Part model, mm, in its own coordinate system. Face numbers are marked on the shaded views. Give positions to 0.01 mm unless a question says otherwise; leave off trailing zeros. Write each loop counter-clockwise with the first axis right and the second up, starting at its lowest first coordinate (ties: lowest second). Pieces come first, ordered by that corner, then holes. Notation, with made-up numbers: (88, 80.25) - (147, 80.25) arc R28 ccw to (147, 118.25) - close; hole circle Ø11 at (63, 16). An arc over 180 degrees is marked (long way). Answer as a JSON object with one key per item and string values. Group by question number.
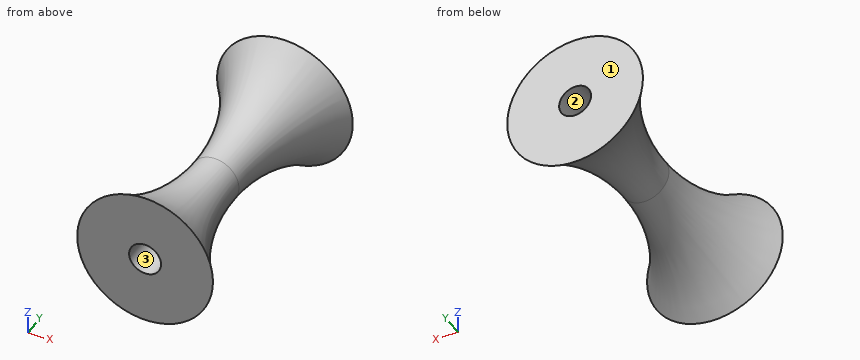
```python
from build123d import *

# Parameters (mm, degrees)
SKETCH1_W          = 3
SKETCH1_H          = 32
SKETCH2_R          = 2
CUT_EXTRUDE1_DEPTH = 35.18332927
CUT_EXTRUDE2_START = -4
SKETCH3_R          = 2.5
CUT_EXTRUDE2_DEPTH = 24
FILLET1_R          = 0.5


with BuildPart() as part:
    # Sketch1 → Revolve1 (revolve)
    with BuildSketch(Plane.XY, mode=Mode.PRIVATE) as revolve1_sk:
        with BuildLine():
            Line((-3, -7e-08), (-3, 16))
            Line((-3, 16), (-8.5, 16))
            ThreePointArc((-8.5, 16), (-4.413382802, 8.459462125), (-3, -7e-08))
        make_face()
        with Locations((-1.5, 0)):
            Rectangle(SKETCH1_W, SKETCH1_H)
        with BuildLine():
            Line((-8.5, -16), (-3, -16))
            Line((-3, -16), (-3, -7e-08))
            ThreePointArc((-3, -7e-08), (-4.413382825, -8.459462191), (-8.5, -16))
        make_face()
    revolve(revolve1_sk.sketch.rotate(Axis((0, 16, 0), (0, -1, 0)), 270), axis=Axis((0, 16, 0), (0, -1, 0)))

    # Sketch2 → Cut-Extrude1 (cut, through all)
    with BuildSketch(Plane(origin=(0, 16, 0), x_dir=(1, 0, 0), z_dir=(0, 1, 0))):
        with Locations(Location((0, 0, 0), (0, 0, 270))):
            Circle(SKETCH2_R)
    extrude(amount=-CUT_EXTRUDE1_DEPTH, mode=Mode.SUBTRACT)

    # Sketch3 → Cut-Extrude2 (cut)
    with BuildSketch(Plane(origin=(0, 16, 0), x_dir=(1, 0, 0), z_dir=(0, 1, 0)).offset(CUT_EXTRUDE2_START)):
        with Locations(Location((0, 0, 0), (0, 0, 270))):
            Circle(SKETCH3_R)
    extrude(amount=-CUT_EXTRUDE2_DEPTH, mode=Mode.SUBTRACT)

    # Fillet1
    fillet1_edges = [part.edges().sort_by_distance(p)[0] for p in [
        (0, 12, -2.5),
        (0, -12, -2.5),
    ]]
    fillet(fillet1_edges, radius=FILLET1_R - 0.0001)  # a hair under: the kernel refuses the full size


solid = part.part
```
1) Saw through at A-A (y = -4). List the corners of the cut face in (x, z), and give its area (3 significant figures).
2) Drill centre lines: line 1 along Y through (x, z) = (0.5, -2); line 2 along Z through (x, y) = (0.75, -4.5); line 3 along Z through (x, y) = (-1.25, 0.5). Where is each one in solid material? Low to high. Write a range as from..to.
3) Drop flat-ended pins along their axis: P1, Ø8, axis at y = -7, z = -2, coming from the -X side; P2, Ø10, axis at y = 0.5, z = -1.5, coming from the -X side; P3, Ø3, axis at x = -3, y = 9.5, coming from the -Z side; P4, Ø3, axis at x = 0, z = 0, coming from the +Y side. Give the stop position or say it passes through.
4) Saw through at B-B (y = -8.5). List the corners of the cut face in (x, z), and give its area (3 significant figures).
5) Two-plate mould, pull along X, no slides. Class the marked faces 1, 2 and 3: +X half, -X half, draft (parallel to the pull), parting line (faces both ways), or undercut.
Checks:
{
 "1": {"outline": "circle Ø6.62 at (0, 0); hole circle Ø5 at (0, 0)", "area": "14.8 mm2"},
 "2": {"line 1": "-16..-12, 12..16", "line 2": "-3.31..-2.38, 2.38..3.31", "line 3": "-2.73..-2.17, 2.17..2.73"},
 "3": {"P1": "x = -5.29", "P2": "x = -3.55", "P3": "z = -4.87", "P4": "through"},
 "4": {"outline": "circle Ø8.85 at (0, 0); hole circle Ø5 at (0, 0)", "area": "41.9 mm2"},
 "5": {"face 1": "draft", "face 2": "undercut", "face 3": "undercut"}
}
